For this review, take the finished solid that the model builds, in its own axes (mm). Face numbers are marked on the shaded views. A direction names the side the tool comes from. Coordinates: 2 decimals unless noted, no trailing zeros. Write each loop counter-clockwise with the first axis right and the second up, starting at its lowest first coordinate (ties: lowest second). Pieces come first, ordered by that corner, then holes.
1) We need section B-B on x = 10. Write out the cut boundary in (y, z).
2) For the marked faces 1, 2 and 3, list the 3-axis set-ups (+Z, -Z, +X, -X, +Y, -Y) from which the entire face can be reached by the end or side of a thin tool; tool diameter is ignored.
3) To check wall thickness, follow line 1 along Y through (x, z) = (10, -26.4); line 2 along Z through (x, y) = (-11, 17.5); line 3 along X through (y, z) = (11, -25.5). State the ranges of each line that lie inside material, in increasing order.
4) We need section A-A on y = 5. Write out the cut boundary in (x, z).
5) Insertion check: P1, Ø1, axis at x = -7.5, y = 12, coming from the +Z side; P2, Ø6.5, axis at x = 10, y = 25, coming from the +Z side; P3, Ø9.5, axis at x = -14, y = 20, coming from the -Z side; P4, Ø10, axis at y = 19, z = -14.5, coming from the +X side. Each pin has a flat end and moves straight along its axis. Give the tip position at first contact, or say it passes through.
6) We need section C-C on y = 28. Write out the cut boundary in (x, z).
7) We need section D-D on z = -10. Write out the cut boundary in (x, y).
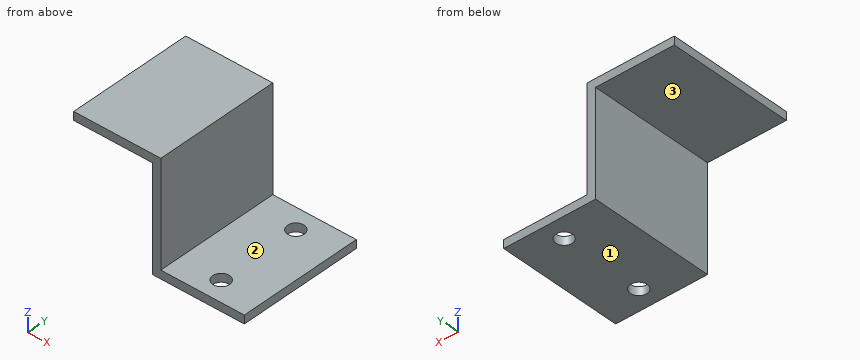
from build123d import *

# Parameters (mm, degrees)
EXTRUDE_1_DEPTH     = 30
SKETCH_2_R          = 2
CUT_EXTRUDE_1_DEPTH = 28


with BuildPart() as part:
    # Эскиз1 → Бобышка-Вытянуть1 (new body)
    with BuildSketch(Plane(origin=(0, 0, 0), x_dir=(1, 0, 0), z_dir=(0, 1, 0))):
        Polygon((0, 0), (-20.856344092, 0), (-20.856344092, 2), (-2, 2), (-2, 27), (20, 27), (20, 25), (0, 25), align=None)
    extrude(amount=EXTRUDE_1_DEPTH)

    # Эскиз2 → Вырез-Вытянуть1 (cut, through all)
    with BuildSketch(Plane(origin=(0, 0, -27), x_dir=(-1, 0, 0), z_dir=(0, 0, -1))):
        with Locations((-10, 25)):
            Circle(SKETCH_2_R)
        with Locations((-10, 5)):
            Circle(SKETCH_2_R)
    extrude(amount=-CUT_EXTRUDE_1_DEPTH, mode=Mode.SUBTRACT)


solid = part.part
Result:
1. outline: (0, -27) - (3, -27) - (3, -25) - (0, -25) - close; (7, -27) - (23, -27) - (23, -25) - (7, -25) - close; (27, -27) - (30, -27) - (30, -25) - (27, -25) - close
2. face 1: -Z, +X, -X, +Y, -Y
2. face 2: +Z, +X, +Y, -Y
2. face 3: -Z, -X, +Y, -Y
3. line 1: y = 0 to 3, 7 to 23, 27 to 30
3. line 2: z = -2 to 0
3. line 3: x = -2 to 20
4. outline: (-20.86, -2) - (-2, -2) - (-2, -27) - (8, -27) - (8, -25) - (0, -25) - (0, 0) - (-20.86, 0) - close; (12, -27) - (20, -27) - (20, -25) - (12, -25) - close
5. P1: stops at z = 0
5. P2: stops at z = -25
5. P3: stops at z = -2
5. P4: stops at x = 0
6. outline: (-20.86, -2) - (-2, -2) - (-2, -27) - (20, -27) - (20, -25) - (0, -25) - (0, 0) - (-20.86, 0) - close
7. outline: (-2, 0) - (0, 0) - (0, 30) - (-2, 30) - close
